Autodesk Inventor part; units mm, degrees
ref_plane "YZ Plane" through (0, 0, 0) normal (1, 0, 0) x (0, 1, 0)
ref_plane "XZ Plane" through (0, 0, 0) normal (0, 1, 0) x (-1, 0, 0)
ref_plane "XY Plane" through (0, 0, 0) normal (0, 0, 1) x (1, 0, 0)
sketch "Sketch1" plane through (0, 0, 0) normal (0, 1, 0) x (-1, 0, 0)
  line L0 (0, 0) -> (46, 0)
  line L1 (46, 0) -> (46, -46)
  line L2 (46, -46) -> (0, -46)
  line L3 (0, -46) -> (0, 0)
  dimension "d0" = 46
  dimension "d1" = 46
extrude "Extrusion1" add sketch "Sketch1" along normal blind 4.5
sketch "Sketch2" plane through (0, 4.5, 0) normal (0, 1, 0) x (1, 0, 0)
  circle A0 centre (-40, 6) radius 3.05
  line L0 (-46, 0) -> (-46, 46)
  line L1 (-46, 0) -> (0, 0)
  circle A1 centre (-40, 40) radius 3.05
  line L2 (0, 46) -> (-46, 46)
  circle A2 centre (-6, 6) radius 3.05
  line L3 (0, 0) -> (0, 46)
  circle A3 centre (-6, 40) radius 3.05
  dimension "d4" = 6.1
  dimension "d5" = 6
  dimension "d6" = 6
  dimension "d7" = 6.1
  dimension "d8" = 6
  dimension "d9" = 6
  dimension "d10" = 6.1
  dimension "d11" = 6
  dimension "d12" = 6
  dimension "d13" = 6.1
  dimension "d16" = 6
  dimension "d17" = 6
extrude "Extrusion2" add sketch "Sketch2" along normal blind 4 contours A0 | A1 | A2 | A3
sketch "Sketch3" plane through (0, 4.5, 0) normal (0, 1, 0) x (1, 0, 0)
  circle A0 centre (-23, 23) radius 12
  point P0 (0, 0)
  dimension "d18" = 24
hole "Hole1" at (-23, 4.5, -23) direction (0, -1, 0) diameter 24 depth 1.5
properties part number "RotatorTop"
Here's how the part is built. I have some questions about the finished solid (model axes, mm). A direction names the side the tool comes from. Coordinates: 2 decimals unless noted, no trailing zeros. Loops run counter-clockwise (first coordinate to the right, second up) from the corner with the lowest first, then second, coordinate; pieces in that order, holes last.
1. For P1, Ø3, axis at x = -11, z = -32, coming from the +Y side; P2, Ø2, axis at y = 7.5, z = -7, coming from the +X side, each with a flat end and sliding along its axis, tell me the tip position at first contact or that it passes through.
2. Imagine slicing it at D-D, the plane x = -23. Please give me the cut outline in (y, z), and give its area (3 significant figures).
3. For faces 1 (the flat face through (-23, 3, -23)), 2 (the flat face through (-23, 0, -23)), which set-ups out of +Z, -Z, +X, -X, +Y, -Y let a thin tool reach every point of the face, with its end or its side?
4. I need wall thicknesses on L1, parallel to Z at x = -23, y = 3.6; L2, parallel to Y at x = -41, z = -29. Which ranges of each line are inside material? Lowest first, please.
5. Imagine slicing it at A-A, the plane x = -6. Please give me the cut outline in (y, z).
6. If we mould it in two halves opening along Z, with no side actions, what happens to faces 3 (the flat face through (-23, 2, -46)), 4 (the cylindrical face through (-37.183, 6.472, -7.168)), 5 (the flat face through (-6, 8.5, -6))? For each: pulls with the +Z half, pulls with the -Z half, needs draft (parallel to the pull), parting line crosses it, or undercut.
7. Imagine slicing it at B-B, the plane y = 3.75. Please give me the cut outline in (x, z).
8. Imagine slicing it at C-C, the plane z = -6. Please give me the cut outline in (x, y), and give its area (3 significant figures).
Taken from the geometry:
1. P1: stops at y = 4.5
1. P2: stops at x = -2.95
2. outline: (0, -46) - (4.5, -46) - (4.5, -35) - (3, -35) - (3, -11) - (4.5, -11) - (4.5, 0) - (0, 0) - close
2. area: 171 mm2
3. face 1: +Y
3. face 2: +Z, -Z, +X, -X, -Y
4. L1: z = -46 to -35, -11 to 0
4. L2: y = 0 to 4.5
5. outline: (0, -46) - (4.5, -46) - (4.5, -43.05) - (8.5, -43.05) - (8.5, -36.95) - (4.5, -36.95) - (4.5, -9.05) - (8.5, -9.05) - (8.5, -2.95) - (4.5, -2.95) - (4.5, 0) - (0, 0) - close
6. face 3: pulls with the -Z half
6. face 4: undercut
6. face 5: needs draft
7. outline: (-46, -46) - (0, -46) - (0, 0) - (-46, 0) - close; hole circle Ø24 at (-23, -23)
8. outline: (-46, 0) - (0, 0) - (0, 4.5) - (-2.95, 4.5) - (-2.95, 8.5) - (-9.05, 8.5) - (-9.05, 4.5) - (-36.95, 4.5) - (-36.95, 8.5) - (-43.05, 8.5) - (-43.05, 4.5) - (-46, 4.5) - close
8. area: 256 mm2
